from build123d import *

# Parameters (mm, degrees)
SKETCH1_W                = 65
SKETCH1_H                = 60
SKETCH1_R                = 11
BOSS_EXTRUDE1_DEPTH      = 20
CUT_EXTRUDE1_DEPTH       = 49.541219597
CUT_EXTRUDE1_DEPTH_BACK  = 49.541219597
M6_TAPPED_HOLE2_D        = 5
LPATTERN2_COUNT          = 2
LPATTERN2_PITCH          = 12.5
MIRROR2_COPY_1_D         = 5
CUT_EXTRUDE2_DEPTH       = 49.541219597
M6_CLEARANCE_HOLE1_D     = 6.4
M6_CLEARANCE_HOLE1_DEPTH = 4
M6_TAPPED_HOLE1_D        = 5
M6_TAPPED_HOLE1_DEPTH    = 10
M6_TAPPED_HOLE1_TIP      = 1.502151548
FILLET1_R                = 2


with BuildPart() as part:
    # Sketch1 → Boss-Extrude1 (new body)
    with BuildSketch(Plane(origin=(0, 0, 0), x_dir=(1, 0, 0), z_dir=(0, 1, 0))):
        Rectangle(SKETCH1_W, SKETCH1_H)
        with Locations(Location((0, 0, 0), (0, 0, 270))):
            Circle(SKETCH1_R, mode=Mode.SUBTRACT)
    extrude(amount=BOSS_EXTRUDE1_DEPTH)

    # Sketch2 → Cut-Extrude1 (cut, two sides: drawn at the far end of the back side and taken through both)
    with BuildSketch(Plane(origin=(0, 20, 0), x_dir=(1, 0, 0), z_dir=(0, 1, 0)).offset(-CUT_EXTRUDE1_DEPTH_BACK)):
        Polygon((188.294375749, 3), (32.5, 3), (-22.5, 3), (-22.5, -3), (32.5, -3), (188.294375749, -3), (499.883127247, -3), (499.883127247, 3), align=None)
    extrude(amount=CUT_EXTRUDE1_DEPTH + CUT_EXTRUDE1_DEPTH_BACK, mode=Mode.SUBTRACT)

    # M6 Tapped Hole2 (through all)
    with Locations(Plane(origin=(0, 20, 0), x_dir=(1, 0, 0), z_dir=(0, 1, 0))):
        with Locations((12.5, -23.5)):
            m6_tapped_hole2 = Hole(M6_TAPPED_HOLE2_D / 2)

    # LPattern2: M6 Tapped Hole2 ×2
    with Locations(*[(i * LPATTERN2_PITCH, 0, 0) for i in range(1, LPATTERN2_COUNT)]):
        add(m6_tapped_hole2, mode=Mode.SUBTRACT)

    # Mirror2: M6 Tapped Hole2 across plane
    add(m6_tapped_hole2.mirror(Plane(origin=(0, 0, 0), x_dir=(0, 0, 1), z_dir=(1, 0, 0))), mode=Mode.SUBTRACT)

    # Mirror2 copy 1 (through all)
    with Locations(Plane(origin=(-12.5, 20, 0), x_dir=(-1, 0, 0), z_dir=(0, 1, 0))):
        with Locations((12.5, 23.5)):
            Hole(MIRROR2_COPY_1_D / 2)

    # Sketch6 → Cut-Extrude2 (cut, through all)
    with BuildSketch(Plane(origin=(0, 20, 0), x_dir=(1, 0, 0), z_dir=(0, 1, 0))):
        with BuildLine():
            Line((-32.5, 7), (-13.266499161, 7))
            ThreePointArc((-13.266499161, 7), (0, 15), (13.266499161, 7))
            Line((13.266499161, 7), (32.5, 7))
            Line((32.5, 7), (32.5, 30))
            Line((32.5, 30), (-32.5, 30))
            Line((-32.5, 30), (-32.5, 7))
        make_face()
    extrude(amount=-CUT_EXTRUDE2_DEPTH, mode=Mode.SUBTRACT)

    # M6 Clearance Hole1
    with Locations(Plane(origin=(0, 0, -7), x_dir=(-1, 0, 0), z_dir=(0, 0, -1))):
        with Locations((-22.883249581, 10)):
            Hole(M6_CLEARANCE_HOLE1_D / 2, depth=M6_CLEARANCE_HOLE1_DEPTH)

    # M6 Tapped Hole1
    with Locations(Plane(origin=(0, 0, 3), x_dir=(-1, 0, 0), z_dir=(0, 0, -1))):
        with Locations((-22.883249581, 10)):
            Hole(M6_TAPPED_HOLE1_D / 2, depth=M6_TAPPED_HOLE1_DEPTH)
            with Locations((0, 0, -(M6_TAPPED_HOLE1_DEPTH + M6_TAPPED_HOLE1_TIP / 2))):  # 118° drill point
                Cone(0, M6_TAPPED_HOLE1_D / 2, M6_TAPPED_HOLE1_TIP, mode=Mode.SUBTRACT)

    # Fillet1
    fillet1_edges = [part.edges().sort_by_distance(p)[0] for p in [
        (-10.583005244, 10, 3),
        (10.583005244, 10, 3),
        (10.583005244, 10, -3),
        (-10.583005244, 10, -3),
        (-22.5, 10, 3),
        (-22.5, 10, -3),
        (32.5, 10, 3),
        (32.5, 10, -3),
        (-32.5, 10, -7),
        (32.5, 10, -7),
        (13.266499161, 10, -7),
        (-13.266499161, 10, -7),
        (32.5, 10, 30),
        (-32.5, 10, 30),
    ]]
    fillet(fillet1_edges, radius=FILLET1_R - 0.0001)  # a hair under: the kernel refuses the full size


solid = part.part
Source: CAD feature listing. Evaluate the final solid. Frame: model axes, mm. A direction names the side the tool comes from. Round coordinates to 2 decimals unless told otherwise and drop trailing zeros. Loops run counter-clockwise (first coordinate to the right, second up) from the corner with the lowest first, then second, coordinate; pieces in that order, holes last. Notation, with made-up numbers: (-34.75, -7) - (-12.75, -7) arc R18 ccw to (-12.75, 22) - close; hole circle Ø8 at (61, 77). An arc over 180 degrees is marked (long way). Write item = value, one per line. Start each with the question number.
(1) Set-up query: faces 4 (the face through (-16, 10, 3)), 5 (the face through (-10.9, 9.86, 3.33)), 6 (the face through (19, 10, -7)). Return all of +Z, -Z, +X, -X, +Y, -Y with unobstructed straight access to the full face (end or side cutting, diameter ignored); none if empty.
(2) Pin query (flat end, axial travel): pin 1 (6 mm diameter, centred on x = 2, y = 7.5, fed in from -Z); pin 2 (6.5 mm diameter, centred on x = 22.88, y = 10, fed in from -Z); pin 3 (8 mm diameter, centred on y = 7.5, z = -0.5, fed in from +X); pin 4 (3 mm diameter, centred on x = 12.5, z = 23.5, fed in from +Y). Return the tip coordinate at first contact, or that it passes through.
(3) Ray query, line 1 along X through (y, z) = (18.25, 24); line 2 along Z through (x, y) = (-25, 8.25); line 3 along Z through (x, y) = (11.5, 6.5). Return the intervals inside material, ascending. Write a range as from..to.
(4) Section query D-D, the plane y = 14.5. State how many separate pieces and enclosed holes the cut face has, plus the area to 3 significant figures.
(5) Section query B-B, the plane x = -25. Output: boundary loops of the cut face in (y, z), plus the area to 3 significant figures.
(6) Section query A-A, the plane z = 23.5. Output: boundary loops of the cut face in (x, y).
(7) Section query C-C, the plane z = 6.5. Output: boundary loops of the cut face in (x, y), plus the area to 3 significant figures.
(8) Pull-direction query (Y, two-part tool) for faces 1 (the face through (0, 0, 12)), 2 (the face through (-23, 10, -7)), 3 (the face through (25.839, 8.774, -4.972)); classes: +Y half, -Y half, draft (parallel to the pull), parting line (faces both ways), or undercut.
Conclusion:
q1.face_4 = +X, +Y, -Y
q1.face_5 = +Y, -Y
q1.face_6 = -Z, +X, +Y, -Y
q2.pin_1 = -15
q2.pin_2 = -7
q2.pin_3 = 32.44
q2.pin_4 = through
q3.line_1 = -32.5..-27.45, -22.55..-14.95, -10.05..10.05, 14.95..22.55, 27.45..32.5
q3.line_2 = -7..21, 26..30
q3.line_3 = -9.63..-3.06, 3.06..21.21, 25.79..30
q4.separate_pieces = 1
q4.enclosed_holes = 4
q4.area = 1,890 mm2
q5.outline = (0, -7) - (20, -7) - (20, 21) - (0, 21) - close; (0, 26) - (20, 26) - (20, 30) - (0, 30) - close
q5.area = 640 mm2
q6.outline = (-32.5, 0) - (-27.5, 0) - (-27.5, 20) - (-32.5, 20) - close; (-22.5, 0) - (-15, 0) - (-15, 20) - (-22.5, 20) - close; (-10, 0) - (10, 0) - (10, 20) - (-10, 20) - close; (15, 0) - (22.5, 0) - (22.5, 20) - (15, 20) - close; (27.5, 0) - (32.5, 0) - (32.5, 20) - (27.5, 20) - close
q7.outline = (-32.5, 0) - (-8.87, 0) - (-8.87, 20) - (-32.5, 20) - close; (8.87, 0) - (32.5, 0) - (32.5, 20) - (8.87, 20) - close; hole circle Ø5 at (22.88, 10)
q7.area = 925 mm2
q8.face_1 = -Y half
q8.face_2 = draft
q8.face_3 = undercut
